```python
from build123d import *

# Parameters (mm, degrees)
BOSS_EXTRUDE1_DEPTH = 5.08
SKETCH3_R           = 1.905
CUT_EXTRUDE1_DEPTH  = 104.255373831
SKETCH4_R           = 1.905
SKETCH4_R_2         = 2.286
CUT_EXTRUDE2_DEPTH  = 104.255373831
CUT_EXTRUDE3_DEPTH  = 104.255373831
SKETCH6_R           = 15.494
SKETCH6_R_2         = 1.7
CUT_EXTRUDE4_DEPTH  = 104.255373831
SKETCH7_W           = 53.34
SKETCH7_H           = 69.85
CUT_EXTRUDE5_DEPTH  = 104.255373831
SKETCH8_W           = 5.838418679
SKETCH8_H           = 5.514062087
CUT_EXTRUDE6_DEPTH  = 104.255373831
CUT_EXTRUDE7_DEPTH  = 3.81


with BuildPart() as part:
    # Sketch1 → Boss-Extrude1 (new body)
    with BuildSketch(Plane(origin=(0, 0, 0), x_dir=(1, 0, 0), z_dir=(0, 1, 0))):
        Polygon((-15.621, -53.34), (15.621, -53.34), (88.265, -53.34), (88.265, 53.34), (-88.265, 53.34), (-88.265, -53.34), align=None)
    extrude(amount=BOSS_EXTRUDE1_DEPTH)

    # Sketch3 → Cut-Extrude1 (cut, through all)
    with BuildSketch(Plane(origin=(0, 5.08, 0), x_dir=(1, 0, 0), z_dir=(0, 1, 0))):
        with Locations(Location((-81.915, 46.99, 0), (0, 0, 270))):
            Circle(SKETCH3_R)
    extrude(amount=-CUT_EXTRUDE1_DEPTH, mode=Mode.SUBTRACT)

    # Sketch4 → Cut-Extrude2 (cut, through all)
    with BuildSketch(Plane(origin=(0, 5.08, 0), x_dir=(1, 0, 0), z_dir=(0, 1, 0))):
        with Locations(Location((81.915, 46.99, 0), (0, 0, 270))):
            Circle(SKETCH4_R)
        with Locations(Location((-81.915, -46.99, 0), (0, 0, 270))):
            Circle(SKETCH4_R)
        with Locations(Location((81.915, -46.99, 0), (0, 0, 270))):
            Circle(SKETCH4_R)
        with Locations(Location((23.495, 40.64, 0), (0, 0, 270))):
            Circle(SKETCH4_R_2)
        with Locations(Location((-23.495, 40.64, 0), (0, 0, 270))):
            Circle(SKETCH4_R_2)
    extrude(amount=-CUT_EXTRUDE2_DEPTH, mode=Mode.SUBTRACT)

    # Sketch5 → Cut-Extrude3 (cut, through all)
    with BuildSketch(Plane.XZ):
        Polygon((-2.54, 27.94), (-2.54, 5.969), (11.811, 5.969), (11.811, 0.127), (14.859, 0.127), (14.859, 5.969), (33.02, 5.969), (33.02, 29.21), (33.02, 31.75), (26.67, 31.75), (26.67, 27.94), (25.80916534, 27.94), (14.859, 27.94), (14.859, 33.782), (11.811, 33.782), (11.811, 27.94), align=None)
    extrude(amount=-CUT_EXTRUDE3_DEPTH, mode=Mode.SUBTRACT)

    # Sketch6 → Cut-Extrude4 (cut, through all)
    with BuildSketch(Plane(origin=(0, 5.08, 0), x_dir=(1, 0, 0), z_dir=(0, 1, 0))):
        with Locations(Location((60.071, 25.146, 0), (0, 0, 270))):
            Circle(SKETCH6_R)
        with Locations(Location((39.9778, 25.146, 0), (0, 0, 270))):
            Circle(SKETCH6_R_2)
        with Locations(Location((80.1642, 25.146, 0), (0, 0, 270))):
            Circle(SKETCH6_R_2)
    extrude(amount=-CUT_EXTRUDE4_DEPTH, mode=Mode.SUBTRACT)

    # Sketch7 → Cut-Extrude5 (cut, through all)
    with BuildSketch(Plane(origin=(0, 5.08, 0), x_dir=(1, 0, 0), z_dir=(0, 1, 0))):
        with Locations((-52.451, -5.715)):
            Rectangle(SKETCH7_W, SKETCH7_H)
    extrude(amount=-CUT_EXTRUDE5_DEPTH, mode=Mode.SUBTRACT)

    # Sketch8 → Cut-Extrude6 (cut, through all)
    with BuildSketch(Plane(origin=(0, 5.08, 0), x_dir=(1, 0, 0), z_dir=(0, 1, 0))):
        with Locations((52.991758435, 3.486833379)):
            Rectangle(SKETCH8_W, SKETCH8_H)
    extrude(amount=-CUT_EXTRUDE6_DEPTH, mode=Mode.SUBTRACT)

    # Sketch9 → Cut-Extrude7 (cut)
    with BuildSketch(Plane(origin=(0, 5.08, 0), x_dir=(1, 0, 0), z_dir=(0, 1, 0))):
        Polygon((29.21, -27.94), (58.42, -27.94), (58.42, -48.26), (32.552533169, -48.26), (-18.161, -48.26), (-18.161, -34.29), (17.399, -34.29), (17.399, -30.48), (24.13, -30.48), (24.13, -34.29), (29.21, -34.29), align=None)
    extrude(amount=-CUT_EXTRUDE7_DEPTH, mode=Mode.SUBTRACT)


solid = part.part
```
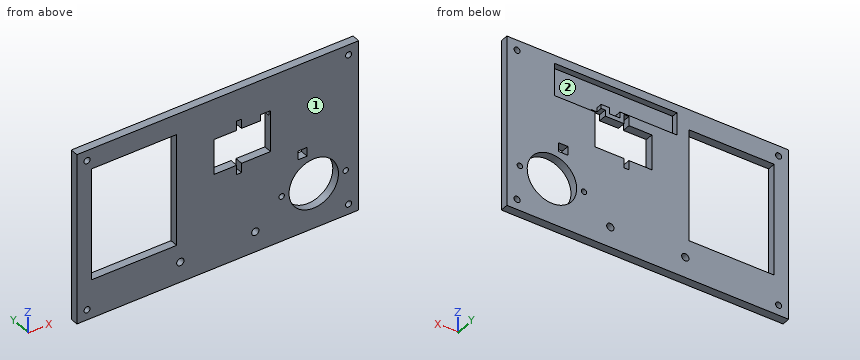
The listing builds one solid part. Answer for the finished solid, in the listing's coordinates (mm). Face numbers are marked on the shaded views. Round coordinates to 2 decimals unless told otherwise and drop trailing zeros. Write each loop counter-clockwise with the first axis right and the second up, starting at its lowest first coordinate (ties: lowest second). Pieces come first, ordered by that corner, then holes. Notation, with made-up numbers: (52.5, 33.25) -> (60.5, 33.25) arc R13 ccw to (60.5, 48.25) -> close; hole circle Ø1 at (30.25, 61.5). An arc over 180 degrees is marked (long way). Use CSV: the item, a comma, the result in double quotes. Start each with the question number.
(1) Consider L1, parallel to X at y = 3.3, z = 21 (3 decimals); L2, parallel to X at y = 3.1, z = -1 (3 decimals); L3, parallel to X at y = 2.4, z = 46.99 (3 decimals). Determine where each line is inside the solid, lowest interval first. Write a range as from..to.
(2) Section A-A on z = -46.99 is taken. Give the vertices of the cut face in (x, y) (3 decimals).
(3) The mould has two halves that part along X. Classify the marked faces 1 and 2: released by +X, released by -X, zero draft, split by the parting line, or undercut.
(4) Each of these flat-tipped pins is pushed along its axis until it touches: pin 1 (3 mm diameter, centred on x = 55.5, z = 36, fed in from +Y); pin 2 (5 mm diameter, centred on x = 81.915, z = 46.99, fed in from +Y). Where does it stop, or does it pass through?
(5) Section D-D on x = -36 is taken. Give the vertices of the cut face in (y, z).
(6) Section C-C on z = -31.5 is taken. Give the vertices of the cut face in (x, y) (3 decimals).
(7) Section B-B on x = 3 is taken. Give the vertices of the cut face in (y, z).
A:
1,L1,"x = -88.265..-79.121, -25.781..-2.54, 33.02..88.265"
1,L2,"x = -88.265..-79.121, -25.781..50.073, 55.911..88.265"
1,L3,"x = -88.265..-83.82, -80.01..-18.161, 58.42..80.01, 83.82..88.265"
2,outline,"(-88.265, 0) -> (-83.82, 0) -> (-83.82, 5.08) -> (-88.265, 5.08) -> close; (-80.01, 0) -> (80.01, 0) -> (80.01, 5.08) -> (-80.01, 5.08) -> close; (83.82, 0) -> (88.265, 0) -> (88.265, 5.08) -> (83.82, 5.08) -> close"
3,face 1,"zero draft"
3,face 2,"undercut"
4,pin 1,"stops at y = 1.27"
4,pin 2,"stops at y = 5.08"
5,outline,"(0, -53.34) -> (5.08, -53.34) -> (5.08, -29.21) -> (0, -29.21) -> close; (0, 40.64) -> (5.08, 40.64) -> (5.08, 53.34) -> (0, 53.34) -> close"
6,outline,"(-88.265, 0) -> (45.94, 0) -> (45.94, 5.08) -> (-88.265, 5.08) -> close; (74.202, 0) -> (88.265, 0) -> (88.265, 5.08) -> (74.202, 5.08) -> close"
7,outline,"(0, -53.34) -> (5.08, -53.34) -> (5.08, 5.97) -> (0, 5.97) -> close; (0, 27.94) -> (5.08, 27.94) -> (5.08, 34.29) -> (1.27, 34.29) -> (1.27, 48.26) -> (5.08, 48.26) -> (5.08, 53.34) -> (0, 53.34) -> close"
